Part model, mm, in its own coordinate system. Face numbers are marked on the shaded views. A direction names the side the tool comes from. Coordinates: 2 decimals unless noted, no trailing zeros. Loops run counter-clockwise (first coordinate to the right, second up) from the corner with the lowest first, then second, coordinate; pieces in that order, holes last. Notation, with made-up numbers: (4.5, 75) -> (19.5, 75) arc R25 ccw to (19.5, 110) -> close; hole circle Ø7 at (-2, -40). An arc over 180 degrees is marked (long way). One line per item, written item: value. Start each with the question number.
from build123d import *

# Parameters (mm, degrees)
SKETCH1_W            = 81.9785
SKETCH1_H            = 52.07
SKETCH1_R            = 1.6129
BASE_PCB_DEPTH       = 1.524
SKETCH2_W            = 6.35
SKETCH2_H            = 6.35
BOSS_EXTRUDE2_DEPTH  = 1.524
SKETCH3_R            = 2.54
BOSS_EXTRUDE3_DEPTH  = 8.128
SKETCH4_W            = 41.0972
SKETCH4_H            = 2.54
LCD_HEADER_DEPTH     = 11.0617
SKETCH5_W            = 80.01
SKETCH5_H            = 36.1315
SKETCH5_R            = 1.6129
LCD_PCB_DEPTH        = 1.524
SKETCH6_W            = 71.374
SKETCH6_H            = 24.13
BOSS_EXTRUDE6_DEPTH  = 7.366
SKETCH7_W            = 65.278
SKETCH7_H            = 13.97
CUT_EXTRUDE1_DEPTH   = 1.27
BOSS_EXTRUDE7_DEPTH  = 3.048
SKETCH9_R            = 6.35
BUZZER_DEPTH         = 6.604
SKETCH10_W           = 5.08
SKETCH10_H           = 17.78
BOSS_EXTRUDE9_DEPTH  = 2.54
SKETCH11_W           = 0.635
SKETCH11_H           = 0.635
BOSS_EXTRUDE10_DEPTH = 6.35
SKETCH12_W           = 5.08
SKETCH12_H           = 7.112
BOSS_EXTRUDE11_DEPTH = 2.54
SKETCH13_W           = 0.635
SKETCH13_H           = 0.635
BOSS_EXTRUDE12_DEPTH = 6.35


with BuildPart() as part:
    # Sketch1 → Base PCB (new body)
    with BuildSketch(Plane(origin=(0, 0, 0), x_dir=(1, 0, 0), z_dir=(0, 1, 0))):
        with Locations((40.98925, -26.035)):
            Rectangle(SKETCH1_W, SKETCH1_H)
        with Locations(Location((3.2639, -4.4069, 0), (0, 0, 90))):
            Circle(SKETCH1_R, mode=Mode.SUBTRACT)
        with Locations(Location((3.2639, -35.5346, 0), (0, 0, 90))):
            Circle(SKETCH1_R, mode=Mode.SUBTRACT)
        with Locations(Location((78.7146, -35.5346, 0), (0, 0, 90))):
            Circle(SKETCH1_R, mode=Mode.SUBTRACT)
        with Locations(Location((78.7146, -4.4069, 0), (0, 0, 90))):
            Circle(SKETCH1_R, mode=Mode.SUBTRACT)
    extrude(amount=BASE_PCB_DEPTH)

    # Sketch2 → Boss-Extrude2 (add)
    with BuildSketch(Plane(origin=(0, 0, 0), x_dir=(-1, 0, 0), z_dir=(0, 0, -1))):
        with Locations((-67.5767, 1.9558)):
            Rectangle(SKETCH2_W, SKETCH2_H)
    extrude(amount=BOSS_EXTRUDE2_DEPTH)

    # Sketch3 → Boss-Extrude3 (add)
    with BuildSketch(Plane(origin=(0, 0, -1.524), x_dir=(-1, 0, 0), z_dir=(0, 0, -1))):
        with Locations((-67.5767, 1.9558)):
            Circle(SKETCH3_R)
    extrude(amount=BOSS_EXTRUDE3_DEPTH)

    # Sketch4 → LCD Header (add)
    with BuildSketch(Plane(origin=(0, 1.524, 0), x_dir=(1, 0, 0), z_dir=(0, 1, 0))):
        with Locations((27.4701, -4.2545)):
            Rectangle(SKETCH4_W, SKETCH4_H)
    extrude(amount=LCD_HEADER_DEPTH)

    # Sketch5 → LCD PCB (add)
    with BuildSketch(Plane(origin=(0, 12.5857, 0), x_dir=(1, 0, 0), z_dir=(0, 1, 0))):
        with Locations((40.98925, -19.97075)):
            Rectangle(SKETCH5_W, SKETCH5_H)
        with Locations(Location((78.7146, -4.4069, 0), (0, 0, 90))):
            Circle(SKETCH5_R, mode=Mode.SUBTRACT)
        with Locations(Location((78.7146, -35.5346, 0), (0, 0, 90))):
            Circle(SKETCH5_R, mode=Mode.SUBTRACT)
        with Locations(Location((3.2639, -35.5346, 0), (0, 0, 90))):
            Circle(SKETCH5_R, mode=Mode.SUBTRACT)
        with Locations(Location((3.2639, -4.4069, 0), (0, 0, 90))):
            Circle(SKETCH5_R, mode=Mode.SUBTRACT)
    extrude(amount=LCD_PCB_DEPTH)

    # Sketch6 → Boss-Extrude6 (add)
    with BuildSketch(Plane(origin=(0, 14.1097, 0), x_dir=(1, 0, 0), z_dir=(0, 1, 0))):
        with Locations((40.90035, -20.447)):
            Rectangle(SKETCH6_W, SKETCH6_H)
    extrude(amount=BOSS_EXTRUDE6_DEPTH)

    # Sketch7 → Cut-Extrude1 (cut)
    with BuildSketch(Plane(origin=(0, 21.4757, 0), x_dir=(1, 0, 0), z_dir=(0, 1, 0))):
        with Locations((40.90035, -20.447)):
            Rectangle(SKETCH7_W, SKETCH7_H)
    extrude(amount=-CUT_EXTRUDE1_DEPTH, mode=Mode.SUBTRACT)

    # Sketch8 → Boss-Extrude7 (add)
    with BuildSketch(Plane(origin=(0, 14.1097, 0), x_dir=(1, 0, 0), z_dir=(0, 1, 0))):
        Polygon((76.58735, -14.732), (76.58735, -26.162), (79.88935, -22.987), (79.88935, -17.907), align=None)
    extrude(amount=BOSS_EXTRUDE7_DEPTH)

    # Sketch9 → Buzzer (add)
    with BuildSketch(Plane(origin=(0, 1.524, 0), x_dir=(1, 0, 0), z_dir=(0, 1, 0))):
        with Locations(Location((6.35, -43.4848, 0), (0, 0, 180))):
            Circle(SKETCH9_R)
    extrude(amount=BUZZER_DEPTH)

    # Sketch10 → Boss-Extrude9 (add)
    with BuildSketch(Plane.XZ):
        with Locations((72.0725, 42.418)):
            Rectangle(SKETCH10_W, SKETCH10_H)
    extrude(amount=BOSS_EXTRUDE9_DEPTH)

    # Sketch11 → Boss-Extrude10 (add)
    with BuildSketch(Plane.ZY.offset(-69.5325)):
        with Locations((37.592, -1.27)):
            Rectangle(SKETCH11_W, SKETCH11_H)
        with Locations((35.179, -1.27)):
            Rectangle(SKETCH11_W, SKETCH11_H)
        with Locations((40.005, -1.27)):
            Rectangle(SKETCH11_W, SKETCH11_H)
        with Locations((42.418, -1.27)):
            Rectangle(SKETCH11_W, SKETCH11_H)
        with Locations((44.831, -1.27)):
            Rectangle(SKETCH11_W, SKETCH11_H)
        with Locations((47.244, -1.27)):
            Rectangle(SKETCH11_W, SKETCH11_H)
        with Locations((49.657, -1.27)):
            Rectangle(SKETCH11_W, SKETCH11_H)
    extrude(amount=BOSS_EXTRUDE10_DEPTH)

    # Sketch12 → Boss-Extrude11 (add)
    with BuildSketch(Plane.XZ):
        with Locations((25.654, 39.37)):
            Rectangle(SKETCH12_W, SKETCH12_H)
    extrude(amount=BOSS_EXTRUDE11_DEPTH)

    # Sketch13 → Boss-Extrude12 (add)
    with BuildSketch(Plane(origin=(28.194, 0, 0), x_dir=(0, 0, -1), z_dir=(1, 0, 0))):
        with Locations((-39.37, -1.27)):
            Rectangle(SKETCH13_W, SKETCH13_H)
        with Locations((-41.783, -1.27)):
            Rectangle(SKETCH13_W, SKETCH13_H)
        with Locations((-36.957, -1.27)):
            Rectangle(SKETCH13_W, SKETCH13_H)
    extrude(amount=BOSS_EXTRUDE12_DEPTH)


solid = part.part
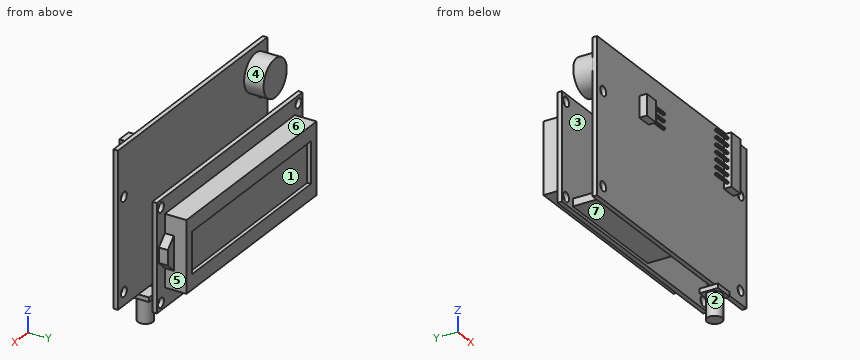
1) Slice it at B-B (z = 12.5). Give the cut face in (x, y).
2) Pin check, flat tips, straight feed: pin 1 Ø1.5 at (y, z) = (16, 20) entering from +X; pin 2 Ø12 at (y, z) = (12, 19) entering from +X; pin 3 Ø0.8 at (y, z) = (-1.5, 39) entering from +X. Stop position of each tip, or through.
3) Probe line 1 (Y direction, x = 58.5, z = 32); line 2 (Y direction, x = 58.5, z = 36.5); line 3 (Z direction, x = 28, y = 2.5). List the from-to ranges inside material, lowest first. Write a range as from..to.
4) Slice it at D-D (z = 4). Give the cut face in (x, y), then the cut area to 3 significant figures.
5) Slice it at A-A (x = 31.5). State how many separate pieces and enclosed holes the cut face has, then the cut area to 3 significant figures.
6) Slice it at C-C (x = 57). Give the cut face in (y, z) (1 decimal), then the cut area to 3 significant figures.
7) Pull direction Y, two halves, no side cores. Call the marked faces 1, 2, 3 and 4: +Y half, -Y half, draft (parallel to the pull), parting line (faces both ways), or undercut.
8) Tool access for the marked faces 5, 6 and 7: list every direction of +Z, -Z, +X, -X, +Y, -Y with a clear straight run to the whole face (end or side of a thin tool).
Check sheet entries:
1. outline: (0, 0) -> (81.98, 0) -> (81.98, 1.52) -> (0, 1.52) -> close; (0.98, 12.59) -> (80.99, 12.59) -> (80.99, 14.11) -> (76.59, 14.11) -> (76.59, 21.48) -> (5.21, 21.48) -> (5.21, 14.11) -> (0.98, 14.11) -> close
2. pin 1: stops at x = 79.89
2. pin 2: stops at x = 80.99
2. pin 3: stops at x = 74.61
3. line 1: y = 0..1.52, 12.59..21.48
3. line 2: y = 0..1.52, 12.59..14.11
3. line 3: z = 2.98..5.52
4. outline: (0, 0) -> (1.7, 0) -> (1.7, 1.52) -> (0, 1.52) -> close; (0.98, 12.59) -> (1.7, 12.59) -> (1.7, 14.11) -> (0.98, 14.11) -> close; (4.82, 0) -> (77.15, 0) -> (77.15, 1.52) -> (48.02, 1.52) -> (48.02, 12.59) -> (77.15, 12.59) -> (77.15, 14.11) -> (4.82, 14.11) -> (4.82, 12.59) -> (6.92, 12.59) -> (6.92, 1.52) -> (4.82, 1.52) -> close; (80.28, 0) -> (81.98, 0) -> (81.98, 1.52) -> (80.28, 1.52) -> close; (80.28, 12.59) -> (80.99, 12.59) -> (80.99, 14.11) -> (80.28, 14.11) -> close
4. area: 682 mm^2
5. separate pieces: 4
5. enclosed holes: 0
5. area: 324 mm^2
6. outline: (0, 0) -> (1.5, 0) -> (1.5, 52.1) -> (0, 52.1) -> close; (12.6, 1.9) -> (14.1, 1.9) -> (14.1, 8.4) -> (21.5, 8.4) -> (21.5, 13.5) -> (20.2, 13.5) -> (20.2, 27.4) -> (21.5, 27.4) -> (21.5, 32.5) -> (14.1, 32.5) -> (14.1, 38) -> (12.6, 38) -> close
6. area: 294 mm^2
7. face 1: +Y half
7. face 2: parting line
7. face 3: undercut
7. face 4: undercut
8. face 5: +X, +Y
8. face 6: +Z, +X, -X, +Y
8. face 7: -Z, +X, -X
